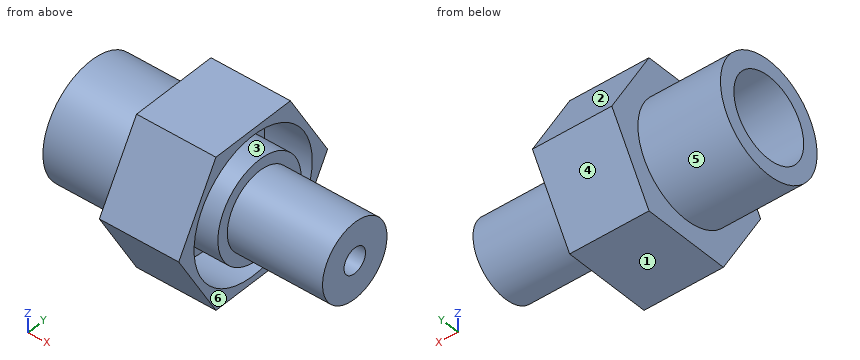
Autodesk Inventor part; units mm, degrees
ref_plane "YZ Plane" through (0, 0, 0) normal (1, 0, 0) x (0, 1, 0)
ref_plane "XZ Plane" through (0, 0, 0) normal (0, 1, 0) x (-1, 0, 0)
ref_plane "XY Plane" through (0, 0, 0) normal (0, 0, 1) x (1, 0, 0)
sketch "Sketch1" plane through (0, 0, 0) normal (0, 0, 1) x (1, 0, 0)
  line L0 (0, 0) -> (-13, 0)
  line L1 (-13, 0) -> (-13, 9)
  line L2 (-13, 9) -> (0, 9)
  line L3 (0, 9) -> (0, 12)
  line L4 (0, 12) -> (12.5, 12)
  line L5 (12.5, 12) -> (12.5, 11)
  line L6 (12.5, 11) -> (5, 11)
  line L7 (5, 11) -> (5, 7.75)
  line L8 (5, 7.75) -> (13.5, 7.75)
  line L9 (13.5, 7.75) -> (13.5, 6)
  line L10 (13.5, 6) -> (28.5, 6)
  line L11 (28.5, 6) -> (28.5, 0)
  line L12 (28.5, 0) -> (0, 0)
  dimension "d0" = 13
  dimension "d1" = 9
  dimension "d2" = 13
  dimension "d3" = 3
  dimension "d4" = 12.5
  dimension "d5" = 1
  dimension "d6" = 7.5
  dimension "d7" = 3.25
  dimension "d8" = 8.5
  dimension "d9" = 1.75
  dimension "d10" = 15
revolve "Revolution1" add sketch "Sketch1" angle 360 about axis through (28.5, 0, 0) along (-1, 0, 0)
sketch "Sketch2" plane through (12.5, 0, 0) normal (1, 0, 0) x (0, 0, -1)
  circle A0 centre (0, 0) radius 12
  line L0 (12, -6.9282) -> (0, -13.8564)
  line L1 (0, -13.8564) -> (-12, -6.9282)
  line L2 (-12, -6.9282) -> (-12, 6.9282)
  line L3 (-12, 6.9282) -> (0, 13.8564)
  line L4 (0, 13.8564) -> (12, 6.9282)
  line L5 (12, 6.9282) -> (12, -6.9282)
  circle A1 centre (0, 0) radius 11
  point P0 (12, 0)
  point P1 (6, 10.3923)
  point P2 (6, -10.3923)
  point P3 (-6, 10.3923)
  point P4 (-12, 0)
  point P5 (-6, -10.3923)
  dimension "d12" = 24
  dimension "d13" = 0
extrude "Extrusion1" add sketch "Sketch2" against normal blind 12.5 contours L5 L0 A0 | A0 L4 L5 | A0 L3 L4 | L0 L1 A0 | A0 L2 L3 | L1 L2 A0
thread "Thread1"
sketch "Sketch3" plane through (-13, 0, 0) normal (-1, 0, 0) x (0, 0, 1)
  circle A0 centre (0, 0) radius 7.75
  circle A1 centre (0, 0) radius 6.5
  dimension "d18" = 13
extrude "Extrusion2" cut sketch "Sketch3" against normal blind 13 contours A1
sketch "Sketch4" plane through (0, 0, 0) normal (-1, 0, 0) x (0, 0, 1)
  circle A0 centre (0, 0) radius 2
  dimension "d21" = 4
extrude "Extrusion3" cut sketch "Sketch4" against normal through all
thread "Thread2"
properties part number "HEX HUB ver 1"
The model under review builds one solid part; all positions refer to its coordinate system, in mm. Face numbers are marked on the shaded views. A direction names the side the tool comes from. Give positions to 0.01 mm unless a question says otherwise; leave off trailing zeros. Write each loop counter-clockwise with the first axis right and the second up, starting at its lowest first coordinate (ties: lowest second). Pieces come first, ordered by that corner, then holes. Notation, with made-up numbers: M -29,30.5 L 8,30.5 A28 cw 8,52.5 Z; hole C 38,-9.75 d1. An arc over 180 degrees is marked long. Write item = value, one per line. Start each with the question number.
Q1. We need section C-C (z = 0.75). State the section outline as (x, y) points, plus the area to 3 significant figures.
Q2. Machinability: for the marked faces 4, 5 and 6, which of the approach directions +Z, -Z, +X, -X, +Y, -Y give a long, thin tool a straight path to every point of the face, cutting with its end or side? Answer none if there is none.
Q3. We need section A-A (x = 2.5). State the section outline as (y, z) points, plus the area to 3 significant figures.
Q4. For line 1 (Y direction, x = 11, z = 0); line 2 (Y direction, x = -6, z = 0); line 3 (X direction, y = 6.75, z = 2), list the stretches that pass through material, from the lowest coordinate up.
Q5. We need section D-D (z = 9.5). State the section outline as (x, y) points, plus the area to 3 significant figures.
Q6. Mouldability with a two-part tool opening along Z and no side actions: class the marked faces 1, 2 and 3 as released by +Z, released by -Z, zero draft, split by the parting line, or undercut.
Q7. We need section B-B (y = 0). State the section outline as (x, z) points, plus the area to 3 significant figures.
Q8. Clearance check with flat-ended pins moving along their axes: pin 1 (10 mm diameter, centred on x = 13.5, y = -6, fed in from +Z); pin 2 (3 mm diameter, centred on x = 18, y = 1.5, fed in from +Z); pin 3 (1 mm diameter, centred on x = -3, y = -11, fed in from +Z); pin 4 (12 mm diameter, centred on x = 19.5, z = -9.5, fed in from +Y). State where each tip first meets the part, or that it passes through.
Result set:
q1.outline = M -13,-8.97 L 0,-8.97 L 0,-13.42 L 12.5,-13.42 L 12.5,-10.97 L 5,-10.97 L 5,-7.71 L 13.5,-7.71 L 13.5,-5.95 L 28.5,-5.95 L 28.5,-1.85 L 0,-1.85 L 0,-6.46 L -13,-6.46 Z; M -13,6.46 L 0,6.46 L 0,1.85 L 28.5,1.85 L 28.5,5.95 L 13.5,5.95 L 13.5,7.71 L 5,7.71 L 5,10.97 L 12.5,10.97 L 12.5,13.42 L 0,13.42 L 0,8.97 L -13,8.97 Z
q1.area = 440 mm2
q2.face_4 = -Z, +X, -X, +Y
q2.face_5 = -X
q2.face_6 = +X
q3.outline = M -13.86,0 L -6.93,-12 L 6.93,-12 L 13.86,0 L 6.93,12 L -6.93,12 Z; hole C 0,0 d4
q3.area = 486 mm2
q4.line_1 = -13.86 to -11, -7.75 to -2, 2 to 7.75, 11 to 13.86
q4.line_2 = -9 to -6.5, 6.5 to 9
q4.line_3 = -13 to 13.5
q5.outline = M 0,-8.37 L 12.5,-8.37 L 12.5,-5.55 L 5,-5.55 L 5,5.55 L 12.5,5.55 L 12.5,8.37 L 0,8.37 Z
q5.area = 126 mm2
q6.face_1 = released by -Z
q6.face_2 = released by +Z
q6.face_3 = undercut
q7.outline = M -13,-9 L 0,-9 L 0,-12 L 12.5,-12 L 12.5,-11 L 5,-11 L 5,-7.75 L 13.5,-7.75 L 13.5,-6 L 28.5,-6 L 28.5,-2 L 0,-2 L 0,-6.5 L -13,-6.5 Z; M -13,6.5 L 0,6.5 L 0,2 L 28.5,2 L 28.5,6 L 13.5,6 L 13.5,7.75 L 5,7.75 L 5,11 L 12.5,11 L 12.5,12 L 0,12 L 0,9 L -13,9 Z
q7.area = 398 mm2
q8.pin_1 = 12
q8.pin_2 = 6
q8.pin_3 = through
q8.pin_4 = 4.87
